from build123d import *

# Parameters (mm, degrees)
F0_W      = 41
F0_H      = 57
F1_DEPTH  = 34
F2_W      = 35
F2_H      = 29
F3_DEPTH  = 57
F4_W      = 3
F4_H      = 5
F4_W_2    = 5
F4_H_2    = 2.5
F5_DEPTH  = 2.5
F6_W      = 35
F6_H      = 2.5
F7_DEPTH  = 47
F8_W      = 24
F8_H      = 12.5
F9_DEPTH  = 41.001
F10_W     = 5
F10_H     = 25
F11_DEPTH = 4
F12_W     = 15
F12_H     = 7
F13_DEPTH = 41.001
F14_DEPTH = 2
F15_W     = 35
F15_H     = 2.25
F16_DEPTH = 5
F17_W     = 3
F17_H     = 5
F17_W_2   = 5
F17_H_2   = 2.5
F18_DEPTH = 2.5


with BuildPart() as f1:
    # F0 (on Top) → F1 (new body)
    with BuildSketch(Plane.XY):
        with Locations((-0.472872518, -12.8149892955)):
            Rectangle(F0_W, F0_H)
    extrude(amount=F1_DEPTH)

    # F2 (on face) → F3 (cut, through all)
    with BuildSketch(Plane.XZ.offset(41.3149892955)):
        with Locations((-0.472872518, 17)):
            Rectangle(F2_W, F2_H)
    extrude(amount=-F3_DEPTH, mode=Mode.SUBTRACT)

    # F4 (on face) → F5 (cut)
    with BuildSketch(Plane(origin=(0, 15.6850107045, 0), x_dir=(-1, 0, 0), z_dir=(0, 1, 0))):
        with Locations((-18.527127482, 17)):
            Rectangle(F4_W, F4_H)
        with Locations((0.472872518, 32.75)):
            Rectangle(F4_W_2, F4_H_2)
        with Locations((19.472872518, 17)):
            Rectangle(F4_W, F4_H)
        with Locations((0.472872518, 1.25)):
            Rectangle(F4_W_2, F4_H_2)
    extrude(amount=-F5_DEPTH, mode=Mode.SUBTRACT)

    # F6 (on face) → F7 (cut)
    with BuildSketch(Plane.XZ.offset(41.3149892955)):
        with Locations((-0.472872518, 32.75)):
            Rectangle(F6_W, F6_H)
    extrude(amount=-F7_DEPTH, mode=Mode.SUBTRACT)

    # F8 (on face) → F9 (cut, through all)
    with BuildSketch(Plane.YZ.offset(20.027127482)):
        with Locations((-1.3149892955, 8.75)):
            Rectangle(F8_W, F8_H)
    extrude(amount=-F9_DEPTH, mode=Mode.SUBTRACT)

    # F10 (on face) → F11 (join)
    with BuildSketch(Plane(origin=(0, 0, 0), x_dir=(1, 0, 0), z_dir=(0, 0, -1))):
        with Locations((17.527127482, 28.8149892955)):
            Rectangle(F10_W, F10_H)
        with Locations((-18.472872518, 28.8149892955)):
            Rectangle(F10_W, F10_H)
    extrude(amount=F11_DEPTH)

    # F12 (on face) → F13 (cut, through all)
    with BuildSketch(Plane.YZ.offset(20.027127482)):
        with Locations((-29.8149892955, 7.5)):
            Rectangle(F12_W, F12_H)
    extrude(amount=-F13_DEPTH, mode=Mode.SUBTRACT)

    # F14 (add): a face of the model
    f14_faces = [f1.faces().sort_by_distance(p)[0] for p in [
        (-0.472872518, 10.5461218156, 31.5),
    ]]
    extrude(f14_faces, amount=F14_DEPTH)

    # F15 (on face) → F16 (join)
    with BuildSketch(Plane.XZ.offset(-5.6850107045)):
        with Locations((-0.472872518, 30.625)):
            Rectangle(F15_W, F15_H)
    extrude(amount=F16_DEPTH)

    # F17 (on face) → F18 (join)
    with BuildSketch(Plane.XZ.offset(41.3149892955)):
        with Locations((18.527127482, 17)):
            Rectangle(F17_W, F17_H)
        with Locations((-19.472872518, 17)):
            Rectangle(F17_W, F17_H)
        with Locations((-0.472872518, 1.25)):
            Rectangle(F17_W_2, F17_H_2)
    extrude(amount=F18_DEPTH)


solid = f1.part
Read the model definition and answer for the solid it produces. Units are mm, in the model's axes. A direction names the side the tool comes from. Give positions to 0.01 mm unless a question says otherwise; leave off trailing zeros. Write each loop counter-clockwise with the first axis right and the second up, starting at its lowest first coordinate (ties: lowest second). Pieces come first, ordered by that corner, then holes. Notation, with made-up numbers: (-5, 68.5) - (36, 68.5) arc R17 cw to (36, 93.5) - close; hole circle Ø11 at (58, 52.5). An arc over 180 degrees is marked (long way). Use CSV: the item, a comma, the result in double quotes. Start each with the question number.
Item 1: The mould has two halves that part along Y. Classify faces 4 (the flat face through (-1, -43.815, 1)), 5 (the flat face through (-19, -13.315, 9)), 6 (the flat face through (-19, 14, 14.5)): pulls with the +Y half, pulls with the -Y half, needs draft (parallel to the pull), parting line crosses it, or undercut.
Item 2: The part is cut by section B-B, the plane x = 9. Give the vertices of the cut face in (y, z), and give its area (3 significant figures).
Item 3: The part is cut by section A-A, the plane y = -29. Give the vertices of the cut face in (x, z).
Item 4: For faces 1 (the flat face through (19, 14, 19.5)), 2 (the flat face through (17.027, -14, 22)), 3 (the flat face through (-2.973, -43, 1)), determine the directions among +Z, -Z, +X, -X, +Y, -Y from which every point of the face is accessible in a straight line to the end or side of a thin tool.
Item 5: The part is cut by section C-C, the plane z = 22. Give the vertices of the cut face in (x, y), and give its area (3 significant figures).
Item 6: Consider line 1 (X direction, y = -28.5, z = 12); line 2 (Z direction, x = 1.5, y = 5); line 3 (Y direction, x = -19, z = 11.5). Determine where each line is inside the solid, lowest interval first.
Item 7: The part is cut by section D-D, the plane z = 30.5. Give the vertices of the cut face in (x, y).
Item 8: Flat-ended cylindrical pins translate along their axes: P1, Ø6, axis at x = -14.5, y = -34, coming from the +Z side; P2, Ø3.5, axis at x = -20, z = 6, coming from the -Y side (3 decimals); P3, Ø0.8, axis at y = -43, z = 1, coming from the -X side. Find the tip coordinate at first contact, or state that the pin passes through.
Taken from the geometry:
1,face 4,"pulls with the -Y half"
1,face 5,"undercut"
1,face 6,"needs draft"
2,outline,"(-41.31, 0) - (15.69, 0) - (15.69, 2.5) - (-41.31, 2.5) - close; (0.69, 29.5) - (15.69, 29.5) - (15.69, 34) - (5.69, 34) - (5.69, 31.75) - (0.69, 31.75) - close"
2,area,"199 mm2"
3,outline,"(-20.97, -4) - (-15.97, -4) - (-15.97, 0) - (15.03, 0) - (15.03, -4) - (20.03, -4) - (20.03, 4) - (17.03, 4) - (17.03, 2.5) - (-17.97, 2.5) - (-17.97, 4) - (-20.97, 4) - close; (-20.97, 11) - (-17.97, 11) - (-17.97, 34) - (-20.97, 34) - close; (17.03, 11) - (20.03, 11) - (20.03, 34) - (17.03, 34) - close"
4,face 1,"+X, -X, +Y"
4,face 2,"-Y"
4,face 3,"+Z, -Z, -X, -Y"
5,outline,"(-20.97, -41.31) - (-17.97, -41.31) - (-17.97, 15.69) - (-20.97, 15.69) - close; (17.03, -41.31) - (20.03, -41.31) - (20.03, 15.69) - (17.03, 15.69) - close"
5,area,"342 mm2"
6,line 1,"-20.97 to -17.97, 17.03 to 20.03"
6,line 2,"0 to 2.5, 29.5 to 31.75"
6,line 3,"-41.31 to -13.31, 10.69 to 15.69"
7,outline,"(-20.97, -41.31) - (-17.97, -41.31) - (-17.97, 0.69) - (17.03, 0.69) - (17.03, -41.31) - (20.03, -41.31) - (20.03, 15.69) - (2.03, 15.69) - (2.03, 13.19) - (-2.97, 13.19) - (-2.97, 15.69) - (-20.97, 15.69) - close"
8,P1,"z = 2.5"
8,P2,"y = -41.315"
8,P3,"x = -2.97"
